Could you check a few things on this model? Use its own coordinates, in mm. A direction names the side the tool comes from. Coordinates: 2 decimals unless noted, no trailing zeros. Write each loop counter-clockwise with the first axis right and the second up, starting at its lowest first coordinate (ties: lowest second). Pieces come first, ordered by that corner, then holes.
```python
from build123d import *

# Parameters (mm, degrees)
FILLET_1_R          = 0.5
FILLET_2_SIZE       = 0.5
FILLET_2_SIZE_2     = 0.8
CHAMFER_1_SIZE      = 0.5
CHAMFER_1_SIZE2     = 0.866025404
CUT_EXTRUDE_1_DEPTH = 3


with BuildPart() as part:
    # 草图2 → 旋转1 (revolve)
    with BuildSketch(Plane(origin=(0, 0, 0), x_dir=(0, 0, -1), z_dir=(1, 0, 0))):
        Polygon((-7.5, 0), (-7.5, 4.9), (-2.5, 4.9), (-2.5, 3), (7.5, 3), (7.5, 0), align=None)
    revolve(axis=Axis((0, 0, -7.5), (0, 0, 1)))

    # 圆角1
    fillet_1_edges = [part.edges().sort_by_distance(p)[0] for p in [
        (0, -4.9, 2.5),
    ]]
    fillet(fillet_1_edges, radius=FILLET_1_R)

    # 圆角2
    # an asymmetric fillet: 0.8, 0.5 mm, written as the material it takes off along each edge
    with BuildSketch(Plane(origin=(0, 0, 7.5), x_dir=(0, 1, 0), z_dir=(1, 0, 0))) as fillet_2_piece_1:
        with BuildLine():
            Bezier((4.9, -FILLET_2_SIZE), (4.9, 0), (4.9 - FILLET_2_SIZE_2, 0), weights=[1, 0.707106781, 1])
            Line((4.9 - FILLET_2_SIZE_2, 0), (4.9, 0))
            Line((4.9, 0), (4.9, -FILLET_2_SIZE))
        make_face()
    revolve(axis=Axis((0, 0, 7.5), (0, 0, 1)), mode=Mode.SUBTRACT)

    # 倒角1
    chamfer_1_edges = [part.edges().sort_by_distance(p)[0] for p in [
        (0, -3, -7.5),
    ]]
    chamfer_1_side = [part.faces().sort_by_distance(p)[0] for p in [
        (0, -3, -2.5),
    ]]
    chamfer(chamfer_1_edges, length=CHAMFER_1_SIZE, length2=CHAMFER_1_SIZE2, reference=chamfer_1_side[0])

    # 草图3 → 切除-拉伸1 (cut)
    with BuildSketch(Plane.XY.offset(7.5)):
        Polygon((0, 2.886751346), (-2.5, 1.443375673), (-2.5, -1.443375673), (0, -2.886751346), (2.5, -1.443375673), (2.5, 1.443375673), align=None)
    extrude(amount=-CUT_EXTRUDE_1_DEPTH, mode=Mode.SUBTRACT)


solid = part.part
```
1. I want a section at A-A on z = -3. Please give me the cut outline in (x, y).
Verdict:
outline: circle Ø6 at (0, 0)
2. Please list where these lines run through material, in increasing order: line 1 along Z through (x, y) = (-1.5, -3.25); line 2 along Z through (x, y) = (1.5, 1.5); line 3 along X through (y, z) = (2.75, 6.5).
Verdict:
line 1: z = 2.5 to 7.5
line 2: z = -7.5 to 4.5
line 3: x = -4.06 to -0.24, 0.24 to 4.06
3. If we mould it in two halves opening along Y, with no side actions, what happens to faces 1 (the face through (0, -3, -2)), 2 (the face through (2.5, 0, 6)), 3 (the face through (0, 0, -7.5))? For each: pulls with the +Y half, pulls with the -Y half, needs draft (parallel to the pull), parting line crosses it, or undercut.
Verdict:
face 1: parting line crosses it
face 2: undercut
face 3: needs draft
4. On a 3-axis mill with a long thin cutter (end or side, diameter ignored), from which of +Z, -Z, +X, -X, +Y, -Y can I reach the whole of each face in a straight line? I mean faces 4 (the face through (2, 2, 7.5)), 5 (the face through (3, 1, 2.5)), 6 (the face through (0, 0, 4.5)). Say none if no direction works.
Verdict:
face 4: +Z, +X, -X, +Y, -Y
face 5: -Z
face 6: +Z
5. For pin 1 (2 mm diameter, centred on x = 0.5, z = 3, fed in from -Y); pin 2 (1.5 mm diameter, centred on x = 0, y = 1.5, fed in from +Z); pin 3 (1.5 mm diameter, centred on x = -2.5, z = 0.5, fed in from -Y); pin 4 (4 mm diameter, centred on y = 1.5, z = -0.5, fed in from +X), each with a flat end and sliding along its axis, tell me the tip position at first contact or that it passes through.
Verdict:
pin 1: stops at y = -4.9
pin 2: stops at z = 4.5
pin 3: stops at y = -2.44
pin 4: stops at x = 3
